```python
from build123d import *

# Parameters (mm, degrees)
F0_W     = 40
F0_H     = 40
F0_R     = 3
F0_R_2   = 11.2
F0_R_3   = 6.15
F1_DEPTH = 2
F2_R     = 5
F3_SIZE  = 1.5


with BuildPart() as f1:
    # F0 (on Top) → F1 (new body)
    with BuildSketch(Plane.XY):
        Rectangle(F0_W, F0_H)
        with Locations((-13.5, -13.5)):
            Circle(F0_R, mode=Mode.SUBTRACT)
        with Locations((13.5, -13.5)):
            Circle(F0_R, mode=Mode.SUBTRACT)
        with Locations((-13.5, 13.5)):
            Circle(F0_R, mode=Mode.SUBTRACT)
        Circle(F0_R_2, mode=Mode.SUBTRACT)
        with Locations((13.5, 13.5)):
            Circle(F0_R, mode=Mode.SUBTRACT)
        Circle(F0_R_2)
        Circle(F0_R_3, mode=Mode.SUBTRACT)
    extrude(amount=F1_DEPTH)

    # F2
    f2_edges = [f1.edges().sort_by_distance(p)[0] for p in [
        (-20, -20, 1),
        (20, -20, 1),
        (20, 20, 1),
        (-20, 20, 1),
    ]]
    fillet(f2_edges, radius=F2_R)

    # F3
    f3_edges = [f1.edges().sort_by_distance(p)[0] for p in [
        (-16.5, 13.5, 2),
        (-16.5, -13.5, 2),
        (10.5, 13.5, 2),
        (10.5, -13.5, 2),
    ]]
    chamfer(f3_edges, length=F3_SIZE)


solid = f1.part
```
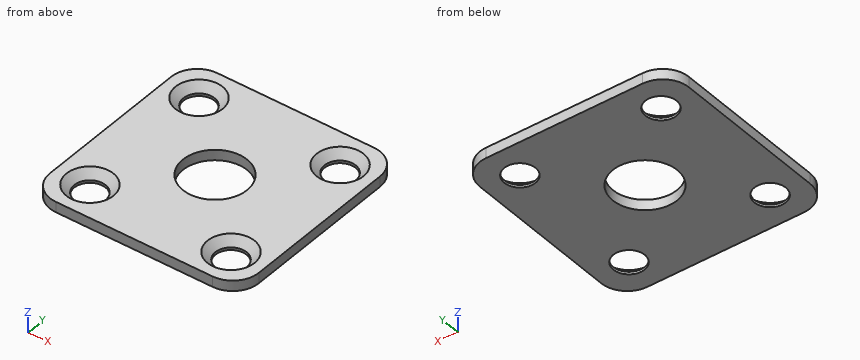
The model under review builds one solid part; all positions refer to its coordinate system, in mm. Coordinates: 2 decimals unless noted, no trailing zeros. Write each loop counter-clockwise with the first axis right and the second up, starting at its lowest first coordinate (ties: lowest second). Pieces come first, ordered by that corner, then holes. Notation, with made-up numbers: (55, 11.5) - (87, 11.5) arc R37 ccw to (87, 49.5) - close; hole circle Ø1 at (-27, 53.25). An arc over 180 degrees is marked (long way). Answer in a Markdown table with one row per item. Add a question column.
Q1. To check wall thickness, follow line 1 along Y through (x, z) = (-13.5, 0.2); line 2 along Y through (x, z) = (0, 0.4); line 3 along X through (y, z) = (-10.5, 1.3). State the ranges of each line that lie inside material, in increasing order. Write a range as from..to.
Q2. Clearance check with flat-ended pins moving along their axes: pin 1 (8 mm diameter, centred on x = -13.5, y = -13.5, fed in from +Z); pin 2 (5 mm diameter, centred on x = 13.5, y = 13.5, fed in from +Z). State where each tip first meets the part, or that it passes through.
Q3. Consider section A-A on y = -13.5. Give the boundary of the cut face in (x, z), then the cut area to 3 significant figures.
Q4. Consider section B-B on z = 1.6. Give the boundary of the cut face in (x, y).
Q5. Consider section C-C on y = 0. Give the boundary of the cut face in (x, z), then the cut area to 3 significant figures.
Answers below:
| question | item | result |
|---|---|---|
| 1 | line 1 | -20..-16.5, -10.5..10.5, 16.5..20 |
| 1 | line 2 | -20..-6.15, 6.15..20 |
| 1 | line 3 | -20..-15.83, -11.17..11.17, 15.83..20 |
| 2 | pin 1 | z = 1.5 |
| 2 | pin 2 | through |
| 3 | outline | (-20, 0) - (-16.5, 0) - (-16.5, 0.5) - (-18, 2) - (-20, 2) - close; (-10.5, 0) - (10.5, 0) - (10.5, 0.5) - (9, 2) - (-9, 2) - (-10.5, 0.5) - close; (16.5, 0) - (20, 0) - (20, 2) - (18, 2) - (16.5, 0.5) - close |
| 3 | area | 51.5 mm² |
| 4 | outline | (-20, -15) arc R5 ccw to (-15, -20) - (15, -20) arc R5 ccw to (20, -15) - (20, 15) arc R5 ccw to (15, 20) - (-15, 20) arc R5 ccw to (-20, 15) - close; hole circle Ø8.2 at (-13.5, -13.5); hole circle Ø8.2 at (-13.5, 13.5); hole circle Ø12.3 at (0, 0); hole circle Ø8.2 at (13.5, -13.5); hole circle Ø8.2 at (13.5, 13.5) |
| 5 | outline | (-20, 0) - (-6.15, 0) - (-6.15, 2) - (-20, 2) - close; (6.15, 0) - (20, 0) - (20, 2) - (6.15, 2) - close |
| 5 | area | 55.4 mm² |
